Part model, mm, in its own coordinate system. A direction names the side the tool comes from. Give positions to 0.01 mm unless a question says otherwise; leave off trailing zeros. Loops run counter-clockwise (first coordinate to the right, second up) from the corner with the lowest first, then second, coordinate; pieces in that order, holes last. Notation, with made-up numbers: (83, 54.5) -> (129, 54.5) arc R26 cw to (129, 71.5) -> close; hole circle Ø10 at (62.5, 17.5). An arc over 180 degrees is marked (long way). Write item = value, one per line.
from build123d import *

# Parameters (mm, degrees)
SKETCH1_W               = 38.1
SKETCH1_H               = 76.2
BOSS_EXTRUDE1_DEPTH     = 76.2
SKETCH2_W               = 6.35
SKETCH2_H               = 50.8
CUT_EXTRUDE1_DEPTH      = 94.3255592
F_1_4_CLEARANCE_HOLE1_D = 6.7564
F_3_8_CLEARANCE_HOLE1_D = 10.0838
SKETCH7_R               = 4.7625
CUT_EXTRUDE2_DEPTH      = 94.325559323


with BuildPart() as part:
    # Sketch1 → Boss-Extrude1 (new body)
    with BuildSketch(Plane(origin=(0, 0, 0), x_dir=(1, 0, 0), z_dir=(0, 1, 0))):
        with Locations((-19.05, 0)):
            Rectangle(SKETCH1_W, SKETCH1_H)
    extrude(amount=BOSS_EXTRUDE1_DEPTH)

    # Sketch2 → Cut-Extrude1 (cut, through all)
    with BuildSketch(Plane(origin=(0, 76.2, 0), x_dir=(1, 0, 0), z_dir=(0, 1, 0))):
        with Locations((-3.175, 0)):
            Rectangle(SKETCH2_W, SKETCH2_H)
    extrude(amount=-CUT_EXTRUDE1_DEPTH, mode=Mode.SUBTRACT)

    # 1/4 Clearance Hole1 (through all)
    with Locations(Plane(origin=(0, 0, 0), x_dir=(0, 0, -1), z_dir=(1, 0, 0))):
        with Locations((0, 50.8), (0, 25.4), (-25.4, 25.4), (-25.4, 50.8), (25.4, 50.8), (25.4, 25.4)):
            Hole(F_1_4_CLEARANCE_HOLE1_D / 2)

    # 3/8 Clearance Hole1 (through all)
    with Locations(Plane(origin=(0, 76.2, 0), x_dir=(1, 0, 0), z_dir=(0, 1, 0))):
        with Locations((-25.4, 0)):
            Hole(F_3_8_CLEARANCE_HOLE1_D / 2)

    # Sketch7 → Cut-Extrude2 (cut, through all)
    with BuildSketch(Plane(origin=(0, 76.2, 0), x_dir=(1, 0, 0), z_dir=(0, 1, 0))):
        with Locations((-6.35, 12.7)):
            Circle(SKETCH7_R)
        with Locations((-6.35, -12.7)):
            Circle(SKETCH7_R)
    extrude(amount=-CUT_EXTRUDE2_DEPTH, mode=Mode.SUBTRACT)


solid = part.part
1) Slice it at C-C, the plane x = -33. List the corners of the cut face in (y, z).
Resolved:
outline = (0, -38.1) -> (76.2, -38.1) -> (76.2, 38.1) -> (0, 38.1) -> close; hole circle Ø6.76 at (25.4, -25.4); hole circle Ø6.76 at (25.4, 0); hole circle Ø6.76 at (25.4, 25.4); hole circle Ø6.76 at (50.8, -25.4); hole circle Ø6.76 at (50.8, 0); hole circle Ø6.76 at (50.8, 25.4)
2) Which spindle directions (+Z, -Z, +X, -X, +Y, -Y) get a long thin tool onto all of the face, cutting with end or side? Do faces 1 (the face through (0, 38, 32)), 2 (the face through (-3, 11, 25.4)). Say none if no direction does.
Resolved:
face_1 = +Z, -Z, +X, +Y, -Y
face_2 = +X, +Y, -Y
3) Slice it at D-D, the plane z = 2. List the corners of the cut face in (x, y), and give its area (3 significant figures).
Resolved:
outline = (-38.1, 0) -> (-30.03, 0) -> (-30.03, 22.68) -> (-38.1, 22.68) -> close; (-38.1, 28.12) -> (-30.03, 28.12) -> (-30.03, 48.08) -> (-38.1, 48.08) -> close; (-38.1, 53.52) -> (-30.03, 53.52) -> (-30.03, 76.2) -> (-38.1, 76.2) -> close; (-20.77, 0) -> (-6.35, 0) -> (-6.35, 22.68) -> (-20.77, 22.68) -> close; (-20.77, 28.12) -> (-6.35, 28.12) -> (-6.35, 48.08) -> (-20.77, 48.08) -> close; (-20.77, 53.52) -> (-6.35, 53.52) -> (-6.35, 76.2) -> (-20.77, 76.2) -> close
area = 1,470 mm²
4) Pull direction Z, two halves, no side cores. Call faces 3 (the face through (-20.363, 37.567, -0.222)), 4 (the face through (-19, 0, -1)), 5 (the face through (-19, 38, -38.1)): pulls with the +Z half, pulls with the -Z half, needs draft (parallel to the pull), parting line crosses it, or undercut.
Resolved:
face_3 = undercut
face_4 = needs draft
face_5 = pulls with the -Z half
5) Drop flat-ended pins along their axis: P1, Ø6.5, axis at y = 23.5, z = 20.5, coming from the +X side; P2, Ø5.5, axis at y = 50.8, z = 0, coming from the -X side; P3, Ø11, axis at y = 50.8, z = -25.4, coming from the +X side. Give the stop position or say it passes through.
Resolved:
P1 = -6.35
P2 = through
P3 = 0
6) Drill centre lines: line 1 along Z through (x, y) = (-35, 25); line 2 along Y through (x, z) = (-28, -25.4); line 3 along Z through (x, y) = (-25.5, 25.4). Where is each one in solid material? Low to high. Write a range as [from, to].
Resolved:
line_1 = [-38.1, -28.75], [-22.05, -3.35], [3.35, 22.05], [28.75, 38.1]
line_2 = [0, 22.02], [28.78, 47.42], [54.18, 76.2]
line_3 = [-38.1, -28.78], [-22.02, -5.04], [5.04, 22.02], [28.78, 38.1]
7) Slice it at A-A, the plane x = -25.4. List the corners of the cut face in (y, z), and give its area (3 significant figures).
Resolved:
outline = (0, -38.1) -> (76.2, -38.1) -> (76.2, -5.04) -> (0, -5.04) -> close; (0, 5.04) -> (76.2, 5.04) -> (76.2, 38.1) -> (0, 38.1) -> close; hole circle Ø6.76 at (25.4, -25.4); hole circle Ø6.76 at (25.4, 25.4); hole circle Ø6.76 at (50.8, -25.4); hole circle Ø6.76 at (50.8, 25.4)
area = 4,890 mm²
8) Slice it at B-B, the plane y = 25.4. Count the separate pieces of the cut face and the enclosed holes in it, and give its area (3 significant figures).
Resolved:
separate_pieces = 4
enclosed_holes = 0
area = 1,810 mm²
